CAD build for the part. Positions are in the model's coordinates, mm. Round coordinates to 2 decimals unless told otherwise and drop trailing zeros. Loops run counter-clockwise (first coordinate to the right, second up) from the corner with the lowest first, then second, coordinate; pieces in that order, holes last.
```python
from build123d import *

# Parameters (mm, degrees)
SKETCH_1_W          = 37
SKETCH_1_H          = 60
EXTRUDE_1_DEPTH     = 3
SKETCH_2_R          = 1.75
CUT_EXTRUDE_1_DEPTH = 3
FILLET_1_R          = 2
SKETCH_3_W          = 25
SKETCH_3_H          = 8
EXTRUDE_2_DEPTH     = 8
FILLET_2_R          = 1
CHAMFER_2_SIZE      = 1
CHAMFER_1_SIZE      = 2


with BuildPart() as part:
    # Эскиз1 → Бобышка-Вытянуть1 (new body)
    with BuildSketch(Plane(origin=(0, 0, 0), x_dir=(1, 0, 0), z_dir=(0, 1, 0))):
        Rectangle(SKETCH_1_W, SKETCH_1_H)
    extrude(amount=EXTRUDE_1_DEPTH)

    # Эскиз2 → Вырез-Вытянуть1 (cut)
    with BuildSketch(Plane(origin=(0, 3, 0), x_dir=(1, 0, 0), z_dir=(0, 1, 0))):
        with Locations(Location((15, 18, 0), (0, 0, 270))):
            Circle(SKETCH_2_R)
        with Locations(Location((15, -18, 0), (0, 0, 90))):
            Circle(SKETCH_2_R)
        with Locations(Location((-15, -18, 0), (0, 0, 270))):
            Circle(SKETCH_2_R)
        with Locations(Location((-15, 18, 0), (0, 0, 90))):
            Circle(SKETCH_2_R)
    extrude(amount=-CUT_EXTRUDE_1_DEPTH, mode=Mode.SUBTRACT)

    # Скругление1
    fillet_1_edges = [part.edges().sort_by_distance(p)[0] for p in [
        (18.5, 1.5, 30),
        (-18.5, 1.5, 30),
        (-18.5, 1.5, -30),
        (18.5, 1.5, -30),
    ]]
    fillet(fillet_1_edges, radius=FILLET_1_R)

    # Эскиз3 → Бобышка-Вытянуть2 (add)
    with BuildSketch(Plane.XZ):
        with Locations((0, 26)):
            Rectangle(SKETCH_3_W, SKETCH_3_H)
    extrude(amount=EXTRUDE_2_DEPTH)

    # Скругление2
    fillet_2_edges = [part.edges().sort_by_distance(p)[0] for p in [
        (12.5, -4, 30),
        (-12.5, -4, 30),
        (0, -8, 30),
    ]]
    fillet(fillet_2_edges, radius=FILLET_2_R)

    # Фаска2
    chamfer_2_edges = [part.edges().sort_by_distance(p)[0] for p in [
        (0, 3, -30),
        (18.5, 3, 0),
        (-18.5, 3, 0),
        (0, 3, 30),
        (17.914213562, 3, 29.414213562),
        (-17.914213562, 3, 29.414213562),
        (-17.914213562, 3, -29.414213562),
        (17.914213562, 3, -29.414213562),
    ]]
    chamfer(chamfer_2_edges, length=CHAMFER_2_SIZE)

    # Фаска1
    # the kernel refuses this chamfer: 2 mm, written as the material it takes off along each edge
    with BuildSketch(Plane(origin=(-15, 3, -18), x_dir=(0, 0, -1), z_dir=(1, 0, 0))) as chamfer_1_piece_1:
        Polygon((1.75 + CHAMFER_1_SIZE, 0), (1.75, -CHAMFER_1_SIZE), (1.75, 0), align=None)
    revolve(axis=Axis((-15, 3, -18), (0, 1, 0)), mode=Mode.SUBTRACT)
    with BuildSketch(Plane(origin=(-15, 3, 18), x_dir=(0, 0, 1), z_dir=(-1, 0, 0))) as chamfer_1_piece_2:
        Polygon((1.75 + CHAMFER_1_SIZE, 0), (1.75, -CHAMFER_1_SIZE), (1.75, 0), align=None)
    revolve(axis=Axis((-15, 3, 18), (0, 1, 0)), mode=Mode.SUBTRACT)
    with BuildSketch(Plane(origin=(15, 3, 18), x_dir=(0, 0, -1), z_dir=(1, 0, 0))) as chamfer_1_piece_3:
        Polygon((1.75 + CHAMFER_1_SIZE, 0), (1.75, -CHAMFER_1_SIZE), (1.75, 0), align=None)
    revolve(axis=Axis((15, 3, 18), (0, 1, 0)), mode=Mode.SUBTRACT)
    with BuildSketch(Plane(origin=(15, 3, -18), x_dir=(0, 0, 1), z_dir=(-1, 0, 0))) as chamfer_1_piece_4:
        Polygon((1.75 + CHAMFER_1_SIZE, 0), (1.75, -CHAMFER_1_SIZE), (1.75, 0), align=None)
    revolve(axis=Axis((15, 3, -18), (0, 1, 0)), mode=Mode.SUBTRACT)


solid = part.part
```
Item 1: Probe line 1 (X direction, y = 0.6, z = -18); line 2 (Y direction, x = -1.5, z = 7.5); line 3 (Z direction, x = 4, y = -4.5). List the from-to ranges inside material, lowest first.
Answers follow:
line 1: x = -18.5 to -16.75, -13.25 to 13.25, 16.75 to 18.5
line 2: y = 0 to 3
line 3: z = 22 to 30
Item 2: Cut at B-B, the plane x = 15. Give the cut face in (y, z).
Answers follow:
outline: (0, -30) - (2, -30) - (3, -29) - (3, -21.75) - (1, -19.75) - (0, -19.75) - close; (0, -16.25) - (1, -16.25) - (3, -14.25) - (3, 14.25) - (1, 16.25) - (0, 16.25) - close; (0, 19.75) - (1, 19.75) - (3, 21.75) - (3, 29) - (2, 30) - (0, 30) - close
Item 3: Cut at C-C, the plane z = -12. Give the cut face in (x, y).
Answers follow:
outline: (-18.5, 0) - (18.5, 0) - (18.5, 2) - (17.5, 3) - (-17.5, 3) - (-18.5, 2) - close
Item 4: Two-plate mould, pull along X, no slides. Class faces 1 (the conical face through (-17.5, 2.6, -28.98)), 2 (the flat face through (0, 0, 0)), 3 (the conical face through (12.95, 1.32, 18.27)), 4 (the conical face through (17.48, 2.6, -29)): released by +X, released by -X, zero draft, split by the parting line, or undercut.
Answers follow:
face 1: released by -X
face 2: zero draft
face 3: undercut
face 4: released by +X
Item 5: Cut at D-D, the plane x = -7. Give the cut face in (y, z), plus the area to 3 significant figures.
Answers follow:
outline: (-8, 22) - (0, 22) - (0, -30) - (2, -30) - (3, -29) - (3, 29) - (2, 30) - (-7, 30) arc R1 ccw to (-8, 29) - close
area: 243 mm2
Item 6: Flat gauge pins, fed straight in: P1, Ø3.5, axis at y = -3, z = 25, coming from the -X side; P2, Ø1.5, axis at x = -2.5, y = -3.5, coming from the -Z side; P3, Ø5.5, axis at x = -15, z = 18, coming from the +Y side; P4, Ø3, axis at x = 15, z = -18, coming from the +Y side. Where does each tip first touch, or does it go through?
Answers follow:
P1: stops at x = -12.5
P2: stops at z = 22
P3: stops at y = 2
P4: passes through
Item 7: Cut at A-A, the plane z = 18. Give the cut face in (x, y) (3 decimals).
Answers follow:
outline: (-18.5, 0) - (-16.75, 0) - (-16.75, 1) - (-18.125, 2.375) - (-18.5, 2) - close; (-13.25, 0) - (13.25, 0) - (13.25, 1) - (11.25, 3) - (-11.25, 3) - (-13.25, 1) - close; (16.75, 0) - (18.5, 0) - (18.5, 2) - (18.125, 2.375) - (16.75, 1) - close
